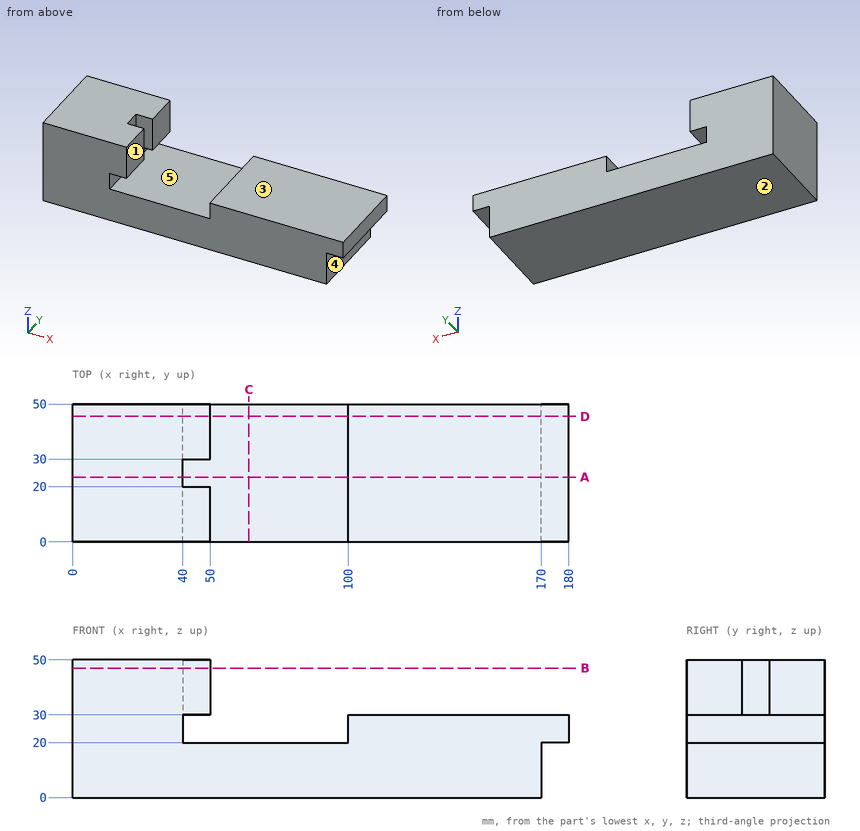
Verification items for this drawing (mm, ordinates from the low corner). A direction names the side the tool comes from. Give positions to 0.01 mm unless a question says otherwise; leave off trailing zeros. Loops run counter-clockwise (first coordinate to the right, second up) from the corner with the lowest first, then second, coordinate; pieces in that order, holes last. Notation, with made-up numbers: M 6,-19 L 60,-19 A27 ccw 60,8 Z; hole C 25.25,27.5 d7. An arc over 180 degrees is marked long. Answer as a JSON object with one key per item and string values. Group by question number.
Item 1: Gauge pin test, flat ends, axial feed: pin 1 (15 mm diameter, centred on x = 80.5, y = 37.5, fed in from +Z); pin 2 (25 mm diameter, centred on x = 141.5, y = 18.5, fed in from +Z); pin 3 (16 mm diameter, centred on y = 26.5, z = 6.5, fed in from +X). Record the tip position at first contact, or that the pin passes through.
Item 2: Sectioned sample at D-D on y = 45.5. Record the boundary of the cut face in (x, z).
Item 3: Mould release check, pull along X, two halves, no side actions. Record for the marked faces 3, 4 and 5: pulls with the +X half, pulls with the -X half, needs draft (parallel to the pull), parting line crosses it, or undercut.
Item 4: Sectioned sample at B-B on z = 47. Record the boundary of the cut face in (x, y), plus the area to 3 significant figures.
Item 5: Access from +Z, -Z, +X, -X, +Y, -Y to the whole of each face (thin tool, end or side, straight path). Record for the marked faces 1 and 2.
Item 6: Material ranges on L1, parallel to X at y = 20.5, z = 11.5; L2, parallel to Z at x = 70.5, y = 34.5; L3, parallel to X at y = 42.5, z = 39.5, recorded low to high.
Item 7: Sectioned sample at C-C on x = 64. Record the boundary of the cut face in (y, z), plus the area to 3 significant figures.
Item 8: Sectioned sample at A-A on y = 23.5. Record the boundary of the cut face in (x, z), plus the area to 3 significant figures.
Findings below:
{
 "1": {"pin 1": "z = 20", "pin 2": "z = 30", "pin 3": "x = 170"},
 "2": {"outline": "M 0,0 L 170,0 L 170,20 L 180,20 L 180,30 L 100,30 L 100,20 L 40,20 L 40,30 L 50,30 L 50,50 L 0,50 Z"},
 "3": {"face 3": "needs draft", "face 4": "pulls with the +X half", "face 5": "undercut"},
 "4": {"outline": "M 0,0 L 50,0 L 50,20 L 40,20 L 40,30 L 50,30 L 50,50 L 0,50 Z", "area": "2,400 mm2"},
 "5": {"face 1": "+Z, +X, +Y, -Y", "face 2": "-Z, +X, -X, +Y, -Y"},
 "6": {"L1": "0 to 170", "L2": "0 to 20", "L3": "0 to 50"},
 "7": {"outline": "M 0,0 L 50,0 L 50,20 L 0,20 Z", "area": "1,000 mm2"},
 "8": {"outline": "M 0,0 L 170,0 L 170,20 L 180,20 L 180,30 L 100,30 L 100,20 L 40,20 L 40,50 L 0,50 Z", "area": "5,400 mm2"}
}
